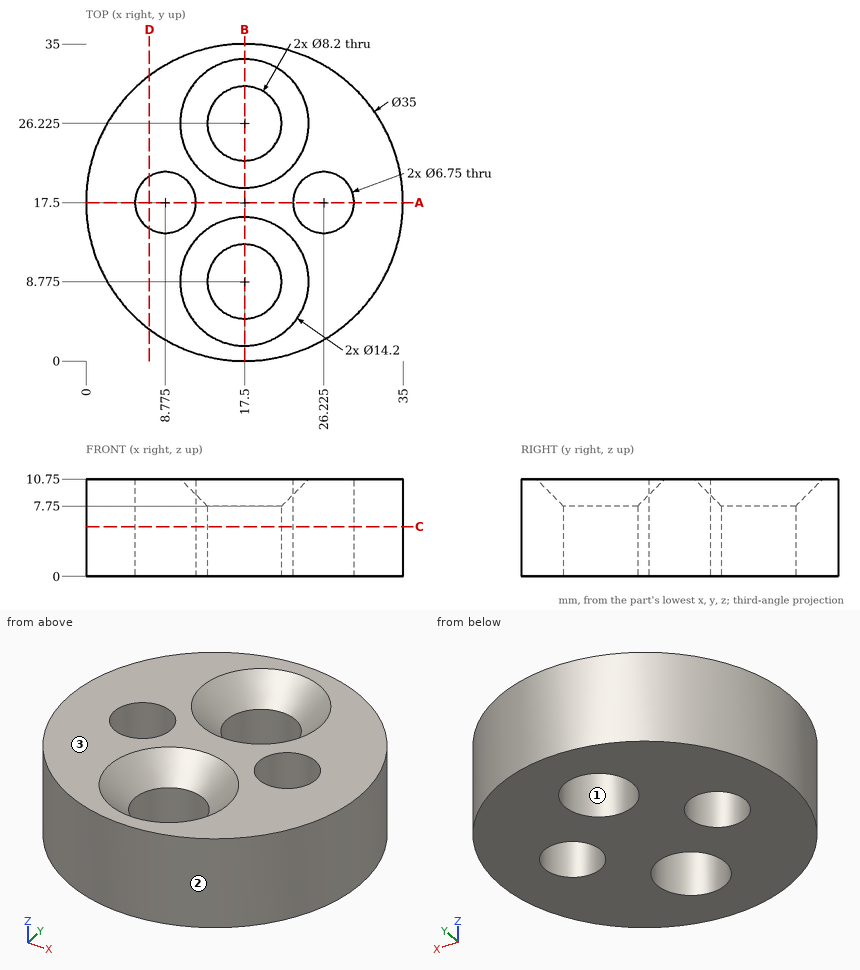
Print and shaded views of the part. All mm, measured from the part's lowest x, y and z. Coordinates: 2 decimals unless noted, no trailing zeros. Order: outer loops, then holes, each group sorted by start corner. A loop starts at its lowest first (then second) coordinate and runs counter-clockwise, first axis right, second up.
(1) Slice it at D-D, the plane x = 7. Write the cut outline in (y, z), and give its area (3 significant figures).
Check sheet entries:
outline: (3.5, 0) - (14.63, 0) - (14.63, 10.75) - (3.5, 10.75) - close; (20.37, 0) - (31.5, 0) - (31.5, 10.75) - (20.37, 10.75) - close
area: 239 mm2
(2) Slice it at B-B, the plane x = 17.5. Write the cut outline in (y, z) (3 decimals).
Check sheet entries:
outline: (0, 0) - (4.675, 0) - (4.675, 7.75) - (1.675, 10.75) - (0, 10.75) - close; (12.875, 0) - (22.125, 0) - (22.125, 7.75) - (19.125, 10.75) - (15.875, 10.75) - (12.875, 7.75) - close; (30.325, 0) - (35, 0) - (35, 10.75) - (33.325, 10.75) - (30.325, 7.75) - close
(3) Probe L1, parallel to Y at x = 17.5, z = 2 (3 decimals); L2, parallel to Y at x = 19, z = 4.25; L3, parallel to X at y = 14.5, z = 6.5. List the from-to ranges inside material, lowest first.
Check sheet entries:
L1: y = 0 to 4.675, 12.875 to 22.125, 30.325 to 35
L2: y = 0.06 to 4.96, 12.59 to 22.41, 30.04 to 34.94
L3: x = 0.26 to 7.23, 10.32 to 24.68, 27.77 to 34.74
(4) Slice it at C-C, the plane z = 5.5. Write the cut outline in (x, y) (3 decimals).
Check sheet entries:
outline: circle Ø35 at (17.5, 17.5); hole circle Ø6.75 at (8.775, 17.5); hole circle Ø8.2 at (17.5, 8.775); hole circle Ø8.2 at (17.5, 26.225); hole circle Ø6.75 at (26.225, 17.5)
(5) Pull direction X, two halves, no side cores. Call the marked faces 1, 2 and 3: pulls with the +X half, pulls with the -X half, needs draft (parallel to the pull), parting line crosses it, or undercut.
Check sheet entries:
face 1: undercut
face 2: parting line crosses it
face 3: needs draft
(6) Slice it at A-A, the plane y = 17.5. Write the cut outline in (x, z).
Check sheet entries:
outline: (0, 0) - (5.4, 0) - (5.4, 10.75) - (0, 10.75) - close; (12.15, 0) - (22.85, 0) - (22.85, 10.75) - (12.15, 10.75) - close; (29.6, 0) - (35, 0) - (35, 10.75) - (29.6, 10.75) - close
(7) Pin check, flat tips, straight feed: pin 1 Ø6.5 at (x, y) = (17.5, 26.225) entering from -Z; pin 2 Ø10.5 at (x, y) = (17.5, 8.775) entering from +Z; pin 3 Ø9 at (x, y) = (8.775, 17.5) entering from -Z; pin 4 Ø1 at (x, z) = (29.5, 9.5) entering from +Y. Stop position of each tip, or through.
Check sheet entries:
pin 1: passes through
pin 2: stops at z = 8.9
pin 3: stops at z = 0
pin 4: stops at y = 30.69
